Design review of the part shown in the three views and the two pictorial views. Dimensions are in mm from the part's minimum x, y and z. Give positions to 0.01 mm unless a question says otherwise; leave off trailing zeros. Write each loop counter-clockwise with the first axis right and the second up, starting at its lowest first coordinate (ties: lowest second). Pieces come first, ordered by that corner, then holes. Notation, with made-up numbers: M 22.25,-22 L 61.25,-22 A17 cw 61.25,-13 Z; hole C 14,0.25 d11. An arc over 180 degrees is marked long. Use one line per item in the form item = value. Start each with the question number.
Q1. Clearance check with flat-ended pins moving along their axes: pin 1 Ø5 at (x, z) = (9.5, 17.5) entering from -Y; pin 2 Ø1.5 at (x, y) = (17.5, 37.5) entering from -Z; pin 3 Ø5 at (y, z) = (56.5, 31) entering from +X; pin 4 Ø12 at (y, z) = (88.5, 27) entering from -X. State where each tip first meets the part, or that it passes through.
Q2. Consider section A-A on x = 11.5. Write out the cut boundary in (y, z), and give its area (3 significant figures).
Q3. Consider section C-C on z = 15. Write out the cut boundary in (x, y), and give its area (3 significant figures).
Q4. Consider section B-B on y = 160. Write out the cut boundary in (x, z).
Q5. For probe 1 along Z at (x, y) = (20, 41.5); probe 2 along X at (y, z) = (127, 18.5); probe 3 along Z at (x, y) = (28.5, 144.5), list the stretches that pass through material, from the lowest coordinate up. Write a range as [from, to].
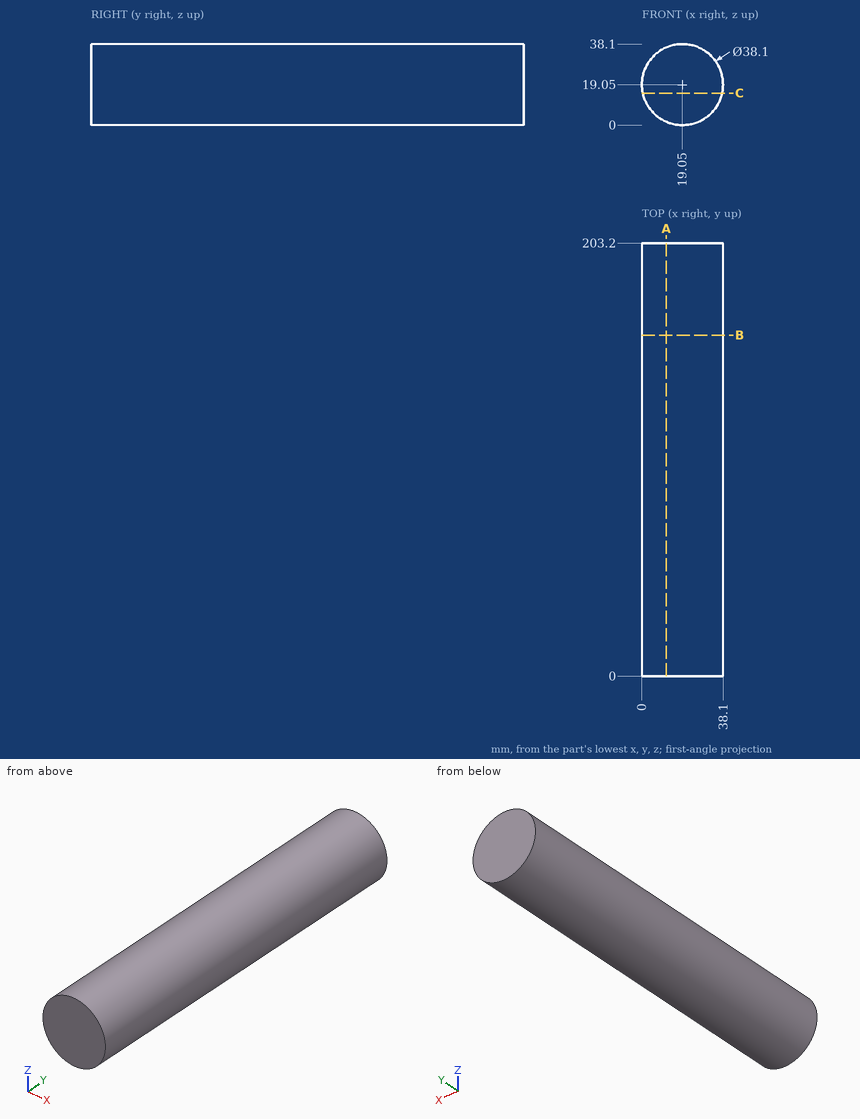
Working result:
q1.pin_1 = 0
q1.pin_2 = 0.02
q1.pin_3 = 35.59
q1.pin_4 = 0.1
q2.outline = M 0,1.56 L 203.2,1.56 L 203.2,36.54 L 0,36.54 Z
q2.area = 7,110 mm²
q3.outline = M 0.44,0 L 37.66,0 L 37.66,203.2 L 0.44,203.2 Z
q3.area = 7,560 mm²
q4.outline = C 19.05,19.05 d38.1
q5.probe_1 = [0.02, 38.08]
q5.probe_2 = [0.01, 38.09]
q5.probe_3 = [2.51, 35.59]
